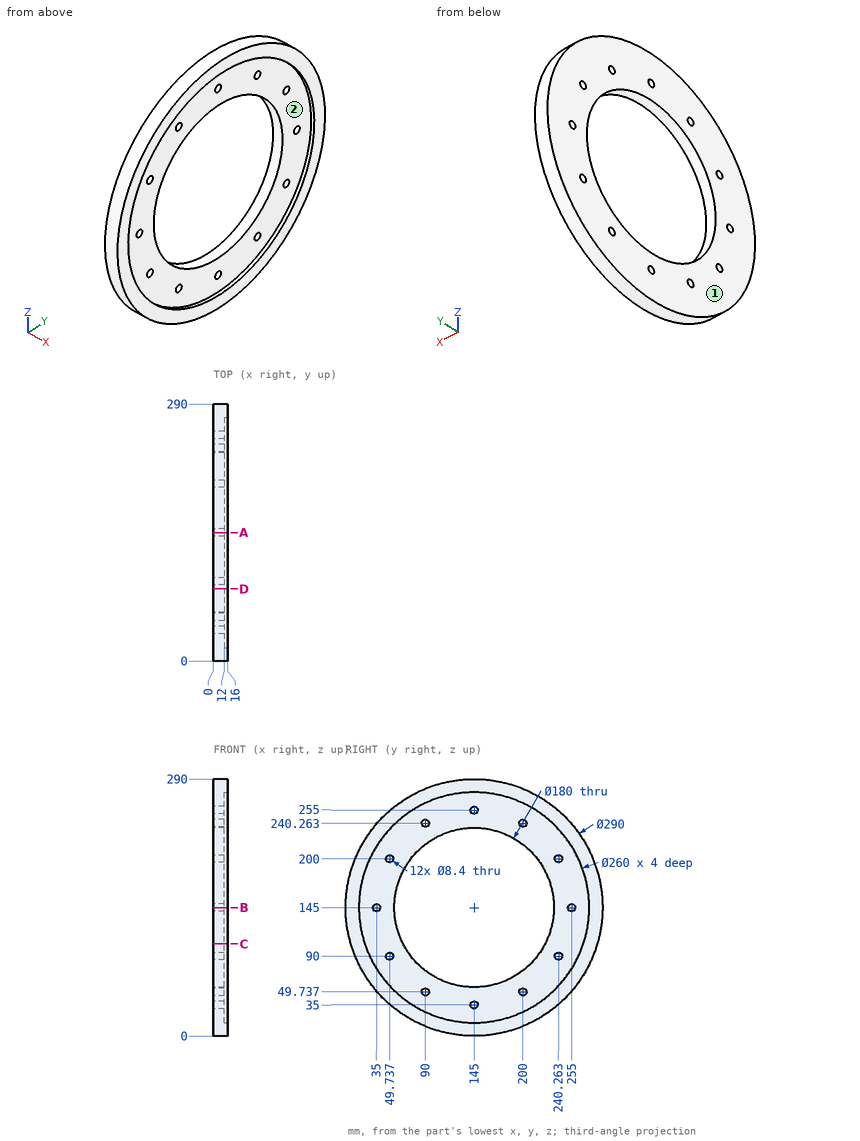
Source: three-view drawing plus pictorial views. Frame: mm from the lowest corner of the part. A direction names the side the tool comes from. Coordinates: 2 decimals unless noted, no trailing zeros. Order: outer loops, then holes, each group sorted by start corner. A loop starts at its lowest first (then second) coordinate and runs counter-clockwise, first axis right, second up.
Item 1: Cut plane A-A (y = 145). Return loops of the section in (x, z).
Output values:
outline: (0, 0) - (16, 0) - (16, 15) - (12, 15) - (12, 30.8) - (0, 30.8) - close; (0, 39.2) - (12, 39.2) - (12, 55) - (0, 55) - close; (0, 235) - (12, 235) - (12, 250.8) - (0, 250.8) - close; (0, 259.2) - (12, 259.2) - (12, 275) - (16, 275) - (16, 290) - (0, 290) - close
Item 2: First-contact query: P1, Ø1.5, axis at x = 12.5, y = 179.5, coming from the -Z side; P2, Ø5, axis at y = 90, z = 49.74, coming from the -X side; P3, Ø9.5, axis at y = 145, z = 35, coming from the +X side; P4, Ø6, axis at x = 8.5, y = 162, coming from the -Z side. Flat tips, straight axial feed; report the tip coordinate or a pass-through.
Output values:
P1: stops at z = 3.98
P2: passes through
P3: stops at x = 12
P4: stops at z = 0.68
Item 3: Set-up query: the marked faces 1 and 2. Return all of +Z, -Z, +X, -X, +Y, -Y with unobstructed straight access to the full face (end or side cutting, diameter ignored); none if empty.
Output values:
face 1: +Z, -Z, -X, +Y, -Y
face 2: +X
Item 4: Material intervals for line 1 (Y direction, x = 4.5, z = 145); line 2 (Y direction, x = 14.95, z = 145); line 3 (X direction, y = 231.5, z = 118), sorted ascending.
Output values:
line 1: y = 0 to 30.8, 39.2 to 55, 235 to 250.8, 259.2 to 290
line 2: y = 0 to 15, 275 to 290
line 3: x = 0 to 12
Item 5: Cut plane D-D (y = 81.5). Return loops of the section in (x, z).
Output values:
outline: (0, 14.64) - (16, 14.64) - (16, 31.56) - (12, 31.56) - (12, 81.22) - (0, 81.22) - close; (0, 208.78) - (12, 208.78) - (12, 258.44) - (16, 258.44) - (16, 275.36) - (0, 275.36) - close
Item 6: Cut plane C-C (z = 104). Return loops of the section in (x, y) (1 decimal), plus the area to 3 significant figures.
Output values:
outline: (0, 5.9) - (16, 5.9) - (16, 21.6) - (12, 21.6) - (12, 64.9) - (0, 64.9) - close; (0, 225.1) - (12, 225.1) - (12, 268.4) - (16, 268.4) - (16, 284.1) - (0, 284.1) - close
area: 1,540 mm2
